from build123d import *

# Parameters (mm, degrees)
SKETCH_1_W          = 40
SKETCH_1_H          = 19.5
SKETCH_1_R          = 1.55
EXTRUDE_1_DEPTH     = 4
CUT_EXTRUDE_1_DEPTH = 4
FILLET_1_R          = 3


with BuildPart() as part:
    # 草图1 → 凸台-拉伸1 (new body)
    with BuildSketch(Plane(origin=(0, 0, 0), x_dir=(1, 0, 0), z_dir=(0, 1, 0))):
        Rectangle(SKETCH_1_W, SKETCH_1_H)
        with Locations(Location((-15, -6.75, 0), (0, 0, 270))):
            Circle(SKETCH_1_R, mode=Mode.SUBTRACT)
        with Locations(Location((-5, -6.75, 0), (0, 0, 270))):
            Circle(SKETCH_1_R, mode=Mode.SUBTRACT)
        with Locations(Location((15, -6.75, 0), (0, 0, 90))):
            Circle(SKETCH_1_R, mode=Mode.SUBTRACT)
        with Locations(Location((5, -6.75, 0), (0, 0, 90))):
            Circle(SKETCH_1_R, mode=Mode.SUBTRACT)
    extrude(amount=EXTRUDE_1_DEPTH)

    # 草图2 → 切除-拉伸1 (cut)
    with BuildSketch(Plane(origin=(0, 4, 0), x_dir=(1, 0, 0), z_dir=(0, 1, 0))):
        with BuildLine():
            Line((-14, 4.25), (14, 4.25))
            ThreePointArc((14, 4.25), (14.707106781, 4.542893219), (15, 5.25))
            Line((15, 5.25), (15, 7.25))
            ThreePointArc((15, 7.25), (14.707106781, 7.957106781), (14, 8.25))
            Line((14, 8.25), (-14, 8.25))
            ThreePointArc((-14, 8.25), (-14.707106781, 7.957106781), (-15, 7.25))
            Line((-15, 7.25), (-15, 5.25))
            ThreePointArc((-15, 5.25), (-14.707106781, 4.542893219), (-14, 4.25))
        make_face()
    extrude(amount=-CUT_EXTRUDE_1_DEPTH, mode=Mode.SUBTRACT)

    # 圆角1
    fillet_1_edges = [part.edges().sort_by_distance(p)[0] for p in [
        (-20, 2, -9.75),
        (20, 2, -9.75),
    ]]
    fillet(fillet_1_edges, radius=FILLET_1_R)


solid = part.part
Build history of the part. All positions in model axes, mm. A direction names the side the tool comes from. Give positions to 0.01 mm unless a question says otherwise; leave off trailing zeros. Loops run counter-clockwise (first coordinate to the right, second up) from the corner with the lowest first, then second, coordinate; pieces in that order, holes last. Notation, with made-up numbers: (59.5, 86) -> (77.5, 86) arc R15 ccw to (77.5, 108) -> close; hole circle Ø9 at (-11.75, 66.5). An arc over 180 degrees is marked (long way). Answer in a Markdown table with one row per item.
Item 1: Probe line 1 along Z through (x, y) = (5, 2.5); line 2 along X through (y, z) = (0.8, 6.75); line 3 along Z through (x, y) = (5.5, 0.8). List the from-to ranges inside material, lowest first. Write a range as [from, to].
Findings below:
| item | result |
|---|---|
| line 1 | z = [-9.75, -8.25], [-4.25, 5.2], [8.3, 9.75] |
| line 2 | x = [-20, -16.55], [-13.45, -6.55], [-3.45, 3.45], [6.55, 13.45], [16.55, 20] |
| line 3 | z = [-9.75, -8.25], [-4.25, 5.28], [8.22, 9.75] |
Item 2: Tool access for faces 1 (the cylindrical face through (19.1, 2.03, -8.89)), 2 (the cylindrical face through (14.699, 2.028, -4.535)): list every direction of +Z, -Z, +X, -X, +Y, -Y with a clear straight run to the whole face (end or side of a thin tool).
Findings below:
| item | result |
|---|---|
| face 1 | -Z, +X, +Y, -Y |
| face 2 | +Y, -Y |
Item 3: Slice it at D-D on x = -5.5. Write the cut outline in (y, z), plus the area to 3 significant figures.
Findings below:
| item | result |
|---|---|
| outline | (0, -9.75) -> (4, -9.75) -> (4, -8.25) -> (0, -8.25) -> close; (0, -4.25) -> (4, -4.25) -> (4, 5.28) -> (0, 5.28) -> close; (0, 8.22) -> (4, 8.22) -> (4, 9.75) -> (0, 9.75) -> close |
| area | 50.3 mm² |
Item 4: Slice it at A-A on x = 11. Write the cut outline in (y, z), plus the area to 3 significant figures.
Findings below:
| item | result |
|---|---|
| outline | (0, -9.75) -> (4, -9.75) -> (4, -8.25) -> (0, -8.25) -> close; (0, -4.25) -> (4, -4.25) -> (4, 9.75) -> (0, 9.75) -> close |
| area | 62.0 mm² |
Item 5: Slice it at B-B on z = 6.75. Write the cut outline in (x, y).
Findings below:
| item | result |
|---|---|
| outline | (-20, 0) -> (-16.55, 0) -> (-16.55, 4) -> (-20, 4) -> close; (-13.45, 0) -> (-6.55, 0) -> (-6.55, 4) -> (-13.45, 4) -> close; (-3.45, 0) -> (3.45, 0) -> (3.45, 4) -> (-3.45, 4) -> close; (6.55, 0) -> (13.45, 0) -> (13.45, 4) -> (6.55, 4) -> close; (16.55, 0) -> (20, 0) -> (20, 4) -> (16.55, 4) -> close |
Item 6: Flat gauge pin, fed straight in: P1, Ø2.5, axis at x = -15, z = 6.75, coming from the -Y side. Where does the tip first touch, or does it go through?
Findings below:
| item | result |
|---|---|
| P1 | passes through |
Item 7: Slice it at C-C on y = 2.8. Write the cut outline in (x, z).
Findings below:
| item | result |
|---|---|
| outline | (-20, -6.75) arc R3 ccw to (-17, -9.75) -> (17, -9.75) arc R3 ccw to (20, -6.75) -> (20, 9.75) -> (-20, 9.75) -> close; hole circle Ø3.1 at (-15, 6.75); hole (-15, -7.25) arc R1 ccw to (-14, -8.25) -> (14, -8.25) arc R1 ccw to (15, -7.25) -> (15, -5.25) arc R1 ccw to (14, -4.25) -> (-14, -4.25) arc R1 ccw to (-15, -5.25) -> close; hole circle Ø3.1 at (-5, 6.75); hole circle Ø3.1 at (5, 6.75); hole circle Ø3.1 at (15, 6.75) |
Item 8: Mould opens along Z. For faces 3 (the cylindrical face through (-13.463, 1.972, 6.548)), 4 (the flat face through (0, 2, -8.25)), 5 (the cylindrical face through (-19.14, 2.03, -8.85)), 6 (the flat face through (-20, 2, 2)) say: pulls with the +Z half, pulls with the -Z half, needs draft (parallel to the pull), parting line crosses it, or undercut.
Findings below:
| item | result |
|---|---|
| face 3 | undercut |
| face 4 | undercut |
| face 5 | pulls with the -Z half |
| face 6 | needs draft |
